```python
from build123d import *

# Parameters (mm, degrees)
F0_W      = 600
F0_H      = 400
F1_DEPTH  = 100
F2_W      = 580
F2_H      = 380
F3_DEPTH  = 80
F4_W      = 400
F4_H      = 50
F5_DEPTH  = 25
F6_W      = 400
F6_H      = 50
F7_DEPTH  = 25
F8_W      = 580
F8_H      = 380
F9_DEPTH  = 20
F10_DEPTH = 400


with BuildPart() as f1:
    # F0 (on Top) → F1 (new body)
    with BuildSketch(Plane.XY):
        Rectangle(F0_W, F0_H)
    extrude(amount=-F1_DEPTH)

    # F2 (on face) → F3 (cut)
    with BuildSketch(Plane(origin=(0, 0, -100), x_dir=(1, 0, 0), z_dir=(0, 0, -1))):
        Rectangle(F2_W, F2_H)
    extrude(amount=-F3_DEPTH, mode=Mode.SUBTRACT)

    # F4 (on face) → F5 (cut)
    with BuildSketch(Plane.XZ.offset(200)):
        with Locations((0, -75)):
            Rectangle(F4_W, F4_H)
    extrude(amount=-F5_DEPTH, mode=Mode.SUBTRACT)

    # F6 (on face) → F7 (cut)
    with BuildSketch(Plane(origin=(0, 200, 0), x_dir=(-1, 0, 0), z_dir=(0, 1, 0))):
        with Locations((0, -75)):
            Rectangle(F6_W, F6_H)
    extrude(amount=-F7_DEPTH, mode=Mode.SUBTRACT)

    # F8 (on face) → F9 (join)
    with BuildSketch(Plane.XY):
        Rectangle(F8_W, F8_H)
    extrude(amount=F9_DEPTH)

    # F10 (add): a face of the model
    f10_faces = [f1.faces().sort_by_distance(p)[0] for p in [
        (0, -200, -37.5),
    ]]
    extrude(f10_faces, amount=-F10_DEPTH)


solid = f1.part
```
The listing builds one solid part. Answer for the finished solid, in the listing's coordinates (mm). A direction names the side the tool comes from. Give positions to 0.01 mm unless a question says otherwise; leave off trailing zeros. Order: outer loops, then holes, each group sorted by start corner. A loop starts at its lowest first (then second) coordinate and runs counter-clockwise, first axis right, second up. Notation, with made-up numbers: (28, 15.25) -> (74, 15.25) arc R37 ccw to (74, 51.25) -> close; hole circle Ø2 at (-35.75, -5.5). An arc over 180 degrees is marked (long way). One line per item, written item: value.
1) Find the intervals of material crossed by line 1 (X direction, y = 134.5, z = -73); line 2 (Z direction, x = 112, y = 162.5); line 3 (X direction, y = -88.5, z = 13.5), in increasing order.
Reported:
line 1: x = -300 to -200, 200 to 300
line 2: z = -50 to 20
line 3: x = -290 to 290
2) A tool of negligible diameter and unlimited length cuts with its end or side. For faces 1 (the flat face through (-4, -190, 10)), 2 (the flat face through (-200, -3, -75)), 3 (the flat face through (-4, 190, 10)), 4 (the flat face through (290, -3, 10)), 5 (the flat face through (-290, -3, 10)), from which of +Z, -Z, +X, -X, +Y, -Y can it reach the whole face along a straight path? Write none if from no direction.
Reported:
face 1: +Z, +X, -X, -Y
face 2: -Z, +Y, -Y
face 3: +Z, +X, -X, +Y
face 4: +Z, +X, +Y, -Y
face 5: +Z, -X, +Y, -Y
3) Find section C-C, the plane y = -38. Determine the outline of the cut face in (x, z), plus the area to 3 significant figures.
Reported:
outline: (-300, -100) -> (-200, -100) -> (-200, -50) -> (200, -50) -> (200, -100) -> (300, -100) -> (300, 0) -> (290, 0) -> (290, 20) -> (-290, 20) -> (-290, 0) -> (-300, 0) -> close
area: 51,600 mm^2
4) Determine the mould class of faces 6 (the flat face through (-251, 3, -100)), 7 (the flat face through (-3, -3, -50)), 8 (the flat face through (300, -3, -49)) for opening direction X: pulls with the +X half, pulls with the -X half, needs draft (parallel to the pull), parting line crosses it, or undercut.
Reported:
face 6: needs draft
face 7: undercut
face 8: pulls with the +X half
5) Flat-ended cylindrical pins translate along their axes: P1, Ø1, axis at x = -119, y = -76, coming from the -Z side; P2, Ø10, axis at x = 223, z = 6, coming from the +Y side; P3, Ø6, axis at y = 86, z = 9.5, coming from the -X side. Find the tip coordinate at first contact, or state that the pin passes through.
Reported:
P1: stops at z = -50
P2: stops at y = 190
P3: stops at x = -290
6) Find section B-B, the plane x = -115. Determine the outline of the cut face in (y, z).
Reported:
outline: (-200, -50) -> (200, -50) -> (200, 0) -> (190, 0) -> (190, 20) -> (-190, 20) -> (-190, 0) -> (-200, 0) -> close
7) Find section A-A, the plane z = -85.5. Determine the outline of the cut face in (x, y).
Reported:
outline: (-300, -200) -> (-200, -200) -> (-200, 200) -> (-300, 200) -> close; (200, -200) -> (300, -200) -> (300, 200) -> (200, 200) -> close
